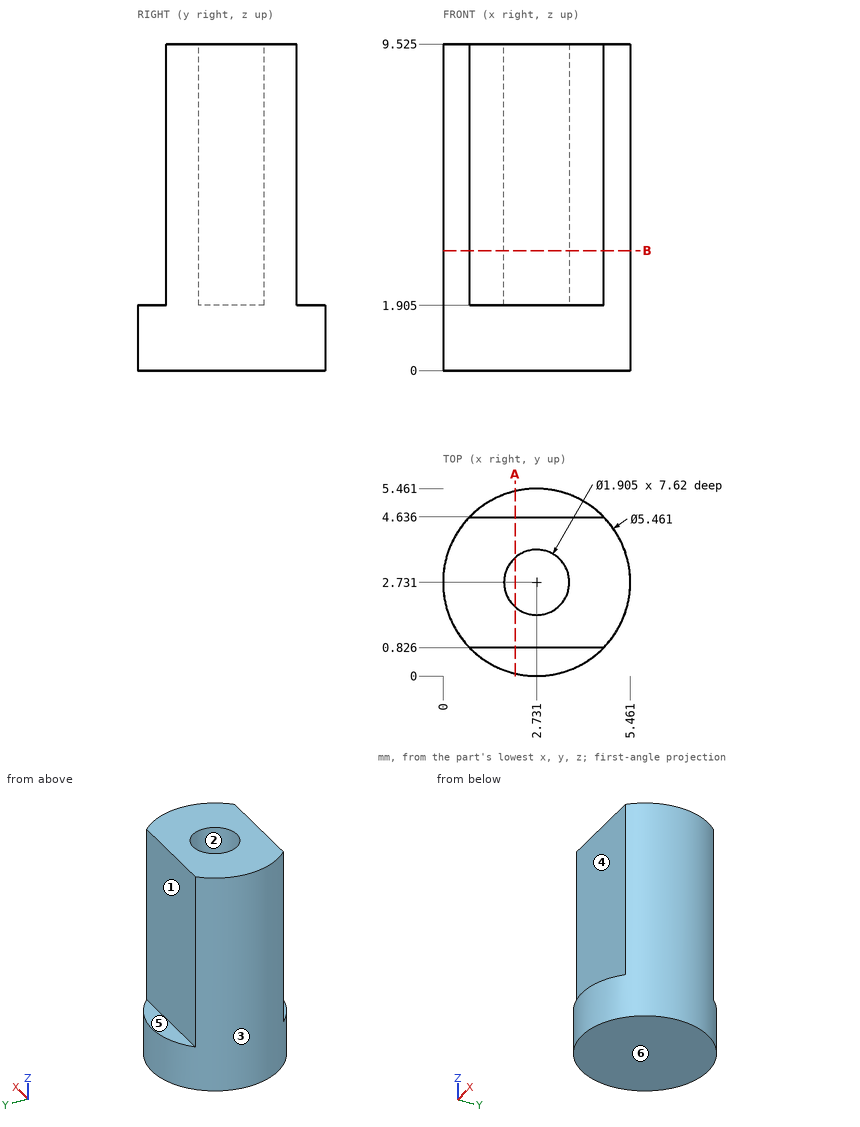
Can you work these out from the drawing? Everything is in mm from the part's minimum corner. A direction names the side the tool comes from. Give positions to 0.01 mm unless a question says otherwise; leave off trailing zeros. Loops run counter-clockwise (first coordinate to the right, second up) from the corner with the lowest first, then second, coordinate; pieces in that order, holes last. Notation, with made-up numbers: M -7.5,-20 L 40.5,-20 A12 ccw 40.5,-6 Z; hole C -25.75,2 d11. An arc over 180 degrees is marked long. Put each result on its own line as item: value. Start each with the question number.
(1) I need wall thicknesses on line 1 along Y through (x, z) = (2.8, 2.75) (1 decimal); line 2 along X through (y, z) = (2.7, 3.75); line 3 along Z through (x, y) = (3.7, 0.3) (1 decimal). Which ranges of each line are inside material? Lowest first, please. Write a range as [from, to].
(2) Will these pins go through, and if not, where does the flat tip stop? pin 1 Ø3 at (y, z) = (1.5, 8.5) entering from +X; pin 2 Ø1.5 at (x, z) = (2, 4) entering from +Y (1 decimal); pin 3 Ø3 at (x, z) = (2, 7.5) entering from -Y (1 decimal); pin 4 Ø1 at (y, z) = (3.5, 1.5) entering from +X.
(3) I want a section at A-A on x = 2.1. Please give me the cut outline in (y, z) (1 decimal).
(4) I want a section at B-B on z = 3.5. Please give me the cut outline in (x, y) (1 decimal).
(5) For the marked faces 4, 5 and 6, which set-ups out of +Z, -Z, +X, -X, +Y, -Y let a thin tool reach every point of the face, with its end or its side?
(6) If we mould it in two halves opening along X, with no side actions, what happens to the marked faces 1, 2 and 3? For each: +X half, -X half, draft (parallel to the pull), parting line (faces both ways), or undercut.
Answer block:
1. line 1: [0.8, 1.8], [3.7, 4.6]
1. line 2: [0, 1.78], [3.68, 5.46]
1. line 3: [0, 1.9]
2. pin 1: x = 5.46
2. pin 2: y = 4.6
2. pin 3: y = 0.8
2. pin 4: x = 5.45
3. outline: M 0.1,0 L 5.4,0 L 5.4,1.9 L 4.6,1.9 L 4.6,9.5 L 3.4,9.5 L 3.4,1.9 L 2,1.9 L 2,9.5 L 0.8,9.5 L 0.8,1.9 L 0.1,1.9 Z
4. outline: M 0.8,0.8 L 4.7,0.8 A2.7 ccw 4.7,4.6 L 0.8,4.6 A2.7 ccw Z; hole C 2.7,2.7 d1.9
5. face 4: +Z, +X, -X, -Y
5. face 5: +Z, +X, -X, +Y
5. face 6: -Z, +X, -X, +Y, -Y
6. face 1: draft
6. face 2: undercut
6. face 3: parting line
